from build123d import *

# Parameters (mm, degrees)
ESBO_O1_W                = 240
ESBO_O1_H                = 160
RESSALTO_EXTRUS_O1_DEPTH = 3
ESBO_O2_W                = 85
ESBO_O2_H                = 45
CORTE_EXTRUS_O1_DEPTH    = 145.25324953
FILETE1_R                = 40
FILETE2_R                = 10


with BuildPart() as part:
    # Esboço1 → Ressalto-extrusão1 (new body)
    with BuildSketch(Plane(origin=(0, 0, 0), x_dir=(1, 0, 0), z_dir=(0, 1, 0))):
        Rectangle(ESBO_O1_W, ESBO_O1_H)
    extrude(amount=RESSALTO_EXTRUS_O1_DEPTH)

    # Esboço2 → Corte-extrusão1 (cut, through all)
    with BuildSketch(Plane(origin=(0, 3, 0), x_dir=(1, 0, 0), z_dir=(0, 1, 0))):
        with Locations((-47.5, -27.5)):
            Rectangle(ESBO_O2_W, ESBO_O2_H)
        with Locations((47.5, 27.5)):
            Rectangle(ESBO_O2_W, ESBO_O2_H)
        with Locations((-47.5, 27.5)):
            Rectangle(ESBO_O2_W, ESBO_O2_H)
        with Locations((47.5, -27.5)):
            Rectangle(ESBO_O2_W, ESBO_O2_H)
    extrude(amount=-CORTE_EXTRUS_O1_DEPTH, mode=Mode.SUBTRACT)

    # Filete1
    filete1_edges = [part.edges().sort_by_distance(p)[0] for p in [
        (-120, 1.5, -80),
        (120, 1.5, -80),
        (120, 1.5, 80),
        (-120, 1.5, 80),
    ]]
    fillet(filete1_edges, radius=FILETE1_R)

    # Filete2
    filete2_edges = [part.edges().sort_by_distance(p)[0] for p in [
        (-90, 1.5, -5),
        (-90, 1.5, -50),
        (-5, 1.5, -50),
        (-5, 1.5, -5),
        (-90, 1.5, 5),
        (-5, 1.5, 5),
        (-5, 1.5, 50),
        (-90, 1.5, 50),
        (90, 1.5, 50),
        (5, 1.5, 50),
        (5, 1.5, 5),
        (90, 1.5, 5),
        (5, 1.5, -50),
        (90, 1.5, -50),
        (90, 1.5, -5),
        (5, 1.5, -5),
    ]]
    fillet(filete2_edges, radius=FILETE2_R)


solid = part.part
CAD build for the part. Positions are in the model's coordinates, mm. A direction names the side the tool comes from. Give positions to 0.01 mm unless a question says otherwise; leave off trailing zeros. Write each loop counter-clockwise with the first axis right and the second up, starting at its lowest first coordinate (ties: lowest second). Pieces come first, ordered by that corner, then holes. Notation, with made-up numbers: M -8.5,72 L 1.5,72 A6 ccw 1.5,81 Z; hole C 66,33.25 d7. An arc over 180 degrees is marked long. Put each result on its own line as item: value. Start each with the question number.
(1) Flat gauge pin, fed straight in: pin 1 Ø1 at (x, y) = (85.5, 2.5) entering from -Z. Where does the tip first touch, or does it go through?
(2) Band-saw the part on B-B, the plane z = -28.5. Write the cut outline in (x, y).
(3) Which spindle directions (+Z, -Z, +X, -X, +Y, -Y) get a long thin tool onto all of the face, cutting with end or side? Do faces 4 (the face through (8.01, 1.48, 47.15)), 5 (the face through (-108.594, 1.521, 67.972)). Say none if no direction does.
(4) Probe L1, parallel to Z at x = -60, y = 0.7; L2, parallel to X at y = 1.85, z = -33.5; L3, parallel to X at y = 1.3, z = 47. List the from-to ranges inside material, lowest first.
(5) Band-saw the part on C-C, the plane y = 2.4. Give the number of separate pieces and of enclosed holes in the cut face, and give its area (3 significant figures).
(6) Mould opens along X. For faces 1 (the face through (8.01, 1.48, -7.85)), 2 (the face through (-108.594, 1.521, -67.972)), 3 (the face through (-2, 0, -1)) say: +X half, -X half, draft (parallel to the pull), parting line (faces both ways), or undercut.
(7) Band-saw the part on A-A, the plane x = -9. Write the cut outline in (y, z), and give its area (3 significant figures).
Response values:
1. pin 1: stops at z = -79.69
2. outline: M -120,0 L -90,0 L -90,3 L -120,3 Z; M -5,0 L 5,0 L 5,3 L -5,3 Z; M 90,0 L 120,0 L 120,3 L 90,3 Z
3. face 4: +Y, -Y
3. face 5: +Z, -X, +Y, -Y
4. L1: z = -80 to -50, -5 to 5, 50 to 80
4. L2: x = -120 to -90, -5 to 5, 90 to 120
4. L3: x = -119.38 to -87.14, -7.86 to 7.86, 87.14 to 119.38
5. separate pieces: 1
5. enclosed holes: 4
5. area: 22,100 mm2
6. face 1: undercut
6. face 2: -X half
6. face 3: draft
7. outline: M 0,-80 L 3,-80 L 3,-48 L 0,-48 Z; M 0,-7 L 3,-7 L 3,7 L 0,7 Z; M 0,48 L 3,48 L 3,80 L 0,80 Z
7. area: 234 mm2
